from build123d import *

# Parameters (mm, degrees)
F0_W     = 38
F0_H     = 62
F1_DEPTH = 20.75
F2_R     = 1.25
F2_R_2   = 7
F3_DEPTH = 3.85
F4_DEPTH = 7.8
F5_DEPTH = 20.751
F6_R     = 11
F6_R_2   = 7
F7_DEPTH = 1
F8_R     = 1.75
F9_DEPTH = 4


with BuildPart() as f1:
    # F0 (on Right) → F1 (new body)
    with BuildSketch(Plane.YZ):
        Rectangle(F0_W, F0_H)
    extrude(amount=F1_DEPTH)

    # F2 (on face) → F3 (cut)
    with BuildSketch(Plane.YZ.offset(20.75)):
        with BuildLine():
            ThreePointArc((-4.48197, 3.728898), (-2.769231, 1.823898), (-0.383414, 2.75684))
            ThreePointArc((-0.383414, 2.75684), (2.480769, 23.959841), (-4.48197, 3.728898))
        make_face()
        with Locations((-2.25, 4.013167)):
            Circle(F2_R, mode=Mode.SUBTRACT)
        with Locations((0, 13.5)):
            Circle(F2_R_2, mode=Mode.SUBTRACT)
    extrude(amount=-F3_DEPTH, mode=Mode.SUBTRACT)

    # F2 (on face) → F4 (cut)
    with BuildSketch(Plane.YZ.offset(20.75)):
        with Locations((-2.25, 4.013167)):
            Circle(F2_R)
        with Locations((8.600429, 25.240833)):
            Circle(F2_R)
    extrude(amount=-F4_DEPTH, mode=Mode.SUBTRACT)

    # F2 (on face) → F5 (cut, through all)
    with BuildSketch(Plane.YZ.offset(20.75)):
        with Locations((0, 13.5)):
            Circle(F2_R_2)
    extrude(amount=-F5_DEPTH, mode=Mode.SUBTRACT)

    # F6 (on face) → F7 (cut)
    with BuildSketch(Plane(origin=(0, 0, 0), x_dir=(0, -1, 0), z_dir=(-1, 0, 0))):
        with Locations((0, 13.5)):
            Circle(F6_R)
        with Locations((0, 13.5)):
            Circle(F6_R_2, mode=Mode.SUBTRACT)
    extrude(amount=-F7_DEPTH, mode=Mode.SUBTRACT)

    # F8 (on face) → F9 (cut)
    with BuildSketch(Plane(origin=(0, 19, 0), x_dir=(-1, 0, 0), z_dir=(0, 1, 0))):
        with Locations((-4.25, 23.25)):
            Circle(F8_R)
        with Locations((-4.25, -14.25)):
            Circle(F8_R)
    extrude(amount=-F9_DEPTH, mode=Mode.SUBTRACT)


solid = f1.part
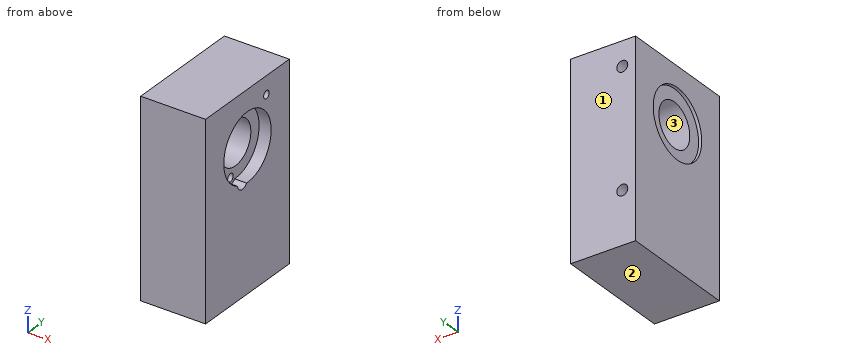
CAD build for the part. Positions are in the model's coordinates, mm. Face numbers are marked on the shaded views. Round coordinates to 2 decimals unless told otherwise and drop trailing zeros. Loops run counter-clockwise (first coordinate to the right, second up) from the corner with the lowest first, then second, coordinate; pieces in that order, holes last. Notation, with made-up numbers: M 84,62 L 89,62 A25 cw 89,79 Z; hole C 82.25,80.25 d7. An arc over 180 degrees is marked long. One line per question, with ' | ' between items. Start each with the question number.
Item 1: Cut at B-B, the plane y = -2.25. Write the cut outline in (x, z), plus the area to 3 significant figures.
Item 2: Wall check: line 1 (Z direction, x = 4.25, y = 17.3); line 2 (Z direction, x = 17.9, y = 0); line 3 (Z direction, x = 5.25, y = 0). Give the ranges that are in metal, low to high.
Item 3: Cut at D-D, the plane z = 11. Write the cut outline in (x, y).
Item 4: Pin check, flat tips, straight feed: pin 1 Ø1 at (x, z) = (3.5, -14) entering from +Y; pin 2 Ø2 at (y, z) = (-2, 5) entering from -X; pin 3 Ø1.5 at (y, z) = (8.6, 25.24) entering from +X. Stop position of each tip, or through.
Item 5: Cut at A-A, the plane x = 12. Write the cut outline in (y, z).
Item 6: Cut at C-C, the plane z = -14.25. Write the cut outline in (x, y).
Item 7: Two-plate mould, pull along Z, no slides. Class the marked faces 1, 2 and 3: pulls with the +Z half, pulls with the -Z half, needs draft (parallel to the pull), parting line crosses it, or undercut.
Responses:
1) outline: M 0,-31 L 20.75,-31 L 20.75,1.76 L 16.9,1.76 L 16.9,2.76 L 12.95,2.76 L 12.95,5.26 L 16.9,5.26 L 16.9,6.87 L 1,6.87 L 1,2.73 L 0,2.73 Z; M 0,24.27 L 1,24.27 L 1,20.13 L 16.9,20.13 L 16.9,24.01 L 20.75,24.01 L 20.75,31 L 0,31 Z | area: 959 mm²
2) line 1: z = -31 to -16, -12.5 to 21.5, 25 to 31 | line 2: z = -31 to 2.75, 24.25 to 31 | line 3: z = -31 to 6.5, 20.5 to 31
3) outline: M 0,-19 L 20.75,-19 L 20.75,-10.46 L 16.9,-10.46 L 16.9,-6.54 L 1,-6.54 L 1,-10.71 L 0,-10.71 Z; M 0,10.71 L 1,10.71 L 1,6.54 L 16.9,6.54 L 16.9,10.46 L 20.75,10.46 L 20.75,19 L 0,19 Z
4) pin 1: stops at y = 15 | pin 2: stops at x = 1 | pin 3: stops at x = 12.95
5) outline: M -19,-31 L 19,-31 L 19,31 L -19,31 Z; hole C 0,13.5 d14
6) outline: M 0,-19 L 20.75,-19 L 20.75,19 L 6,19 L 6,15 L 2.5,15 L 2.5,19 L 0,19 Z
7) face 1: needs draft | face 2: pulls with the -Z half | face 3: undercut
